```python
from build123d import *

# Parameters (mm, degrees)
SKETCH_W      = 51
SKETCH_H      = 56
PAD_DEPTH     = 3
SKETCH001_W   = 51
SKETCH001_H   = 56
SKETCH001_W_2 = 45
SKETCH001_H_2 = 50
PAD001_DEPTH  = 35
SKETCH002_W   = 20
SKETCH002_H   = 35
POCKET_DEPTH  = 3


with BuildPart() as part:
    # Sketch → Pad (new body)
    with BuildSketch(Plane.XY):
        Rectangle(SKETCH_W, SKETCH_H)
    extrude(amount=PAD_DEPTH)

    # Sketch001 (on Face6 of Pad) → Pad001 (join)
    with BuildSketch(Plane.XY.offset(3)):
        Rectangle(SKETCH001_W, SKETCH001_H)
        Rectangle(SKETCH001_W_2, SKETCH001_H_2, mode=Mode.SUBTRACT)
    extrude(amount=PAD001_DEPTH)

    # Sketch002 (on Face10 of Pad001) → Pocket (cut)
    with BuildSketch(Plane.XZ.offset(28)):
        with Locations((0, 20.5)):
            Rectangle(SKETCH002_W, SKETCH002_H)
    extrude(amount=-POCKET_DEPTH, mode=Mode.SUBTRACT)


solid = part.part
```
Source: CAD feature listing. Evaluate the final solid. Frame: model axes, mm. A direction names the side the tool comes from. Round coordinates to 2 decimals unless told otherwise and drop trailing zeros. Loops run counter-clockwise (first coordinate to the right, second up) from the corner with the lowest first, then second, coordinate; pieces in that order, holes last. Notation, with made-up numbers: M -20,37 L 3,37 A26 ccw 3,52 Z; hole C 36.5,39 d10. An arc over 180 degrees is marked long. Use a Markdown table: item, result. Add a question column.
1. Contact query for a flat-ended pin moving along its axis: P1, Ø13.5, axis at x = 1.5, y = 3.5, coming from the +Z side. Output: stop coordinate, or through.
2. Line query: line 1 (Y direction, x = 21.5, z = 20); line 2 (X direction, y = -16, z = 25); line 3 (Z direction, x = 22, y = -14.5). Output: solid intervals per line, ascending.
3. Section query D-D on x = 8. Return the cut outline in (y, z).
4. Section query C-C on z = 29. Return the cut outline in (x, y).
5. Section query A-A on x = 19. Return the cut outline in (y, z), then the cut area to 3 significant figures.
6. Section query B-B on y = -8. Return the cut outline in (x, z), then the cut area to 3 significant figures.
7. Reachability of faces 1 (the flat face through (-10, -27, 20)), 2 (the flat face through (-25.5, 0, 19)), 3 (the flat face through (-22.5, 0, 20)) from +Z, -Z, +X, -X, +Y, -Y: full face, straight path, thin tool, end or side. Return the list, or none.
8. Mould query, pull axis X, two halves, no side actions, for faces 4 (the flat face through (22.5, 0, 20)), 5 (the flat face through (25.5, 0, 19)), 6 (the flat face through (-16, -25, 20)), 7 (the flat face through (0, 0, 0)). Classes: pulls with the +X half, pulls with the -X half, needs draft (parallel to the pull), parting line crosses it, or undercut.
Reported:
| question | item | result |
|---|---|---|
| 1 | P1 | stops at z = 3 |
| 2 | line 1 | y = -28 to -25, 25 to 28 |
| 2 | line 2 | x = -25.5 to -22.5, 22.5 to 25.5 |
| 2 | line 3 | z = 0 to 3 |
| 3 | outline | M -28,0 L 28,0 L 28,38 L 25,38 L 25,3 L -28,3 Z |
| 4 | outline | M -25.5,-28 L -10,-28 L -10,-25 L -22.5,-25 L -22.5,25 L 22.5,25 L 22.5,-25 L 10,-25 L 10,-28 L 25.5,-28 L 25.5,28 L -25.5,28 Z |
| 5 | outline | M -28,0 L 28,0 L 28,38 L 25,38 L 25,3 L -25,3 L -25,38 L -28,38 Z |
| 5 | area | 378 mm² |
| 6 | outline | M -25.5,0 L 25.5,0 L 25.5,38 L 22.5,38 L 22.5,3 L -22.5,3 L -22.5,38 L -25.5,38 Z |
| 6 | area | 363 mm² |
| 7 | face 1 | +Z, -Y |
| 7 | face 2 | +Z, -Z, -X, +Y, -Y |
| 7 | face 3 | +Z |
| 8 | face 4 | undercut |
| 8 | face 5 | pulls with the +X half |
| 8 | face 6 | undercut |
| 8 | face 7 | needs draft |
